The model under review builds one solid part; all positions refer to its coordinate system, in mm. Round coordinates to 2 decimals unless told otherwise and drop trailing zeros. Order: outer loops, then holes, each group sorted by start corner. A loop starts at its lowest first (then second) coordinate and runs counter-clockwise, first axis right, second up. Notation, with made-up numbers: (50, 34.25) -> (69, 34.25) arc R25 ccw to (69, 48.25) -> close; hole circle Ø3 at (37.5, -13.75). An arc over 180 degrees is marked (long way). Put each result on its own line as item: value. Start each with the question number.
Autodesk Inventor part; units mm, degrees
ref_plane "YZ Plane" through (0, 0, 0) normal (1, 0, 0) x (0, 1, 0)
ref_plane "XZ Plane" through (0, 0, 0) normal (0, 1, 0) x (-1, 0, 0)
ref_plane "XY Plane" through (0, 0, 0) normal (0, 0, 1) x (1, 0, 0)
sketch "Эскиз1" plane through (0, 0, 0) normal (0, 0, 1) x (1, 0, 0)
  line L0 (-40, 0) -> (40, 0) construction
  line L1 (-40, -15) -> (40, -15)
  line L2 (40, 15) -> (-40, 15)
  arc A0 (-40, 15) -> (-40, -15) centre (-40, 0) ccw
  arc A1 (40, -15) -> (40, 15) centre (40, 0) ccw
  circle A2 centre (0, 0) radius 12.5
  circle A3 centre (0, 0) radius 6
  circle A4 centre (40, 0) radius 5
  circle A5 centre (-40, 0) radius 5
  dimension "d2" = 80
  dimension "d3" = 30
  dimension "d4" = 25
  dimension "d5" = 12
  dimension "d6" = 10
  dimension "d7" = 10
extrude "Выдавливание1" add sketch "Эскиз1" along normal blind 8 contours A0 L2 A1 L1 | A2 | A4 | A5
extrude "Выдавливание2" cut sketch "Эскиз1" along normal blind 8 contours A4 | A5
extrude "Выдавливание3" add sketch "Эскиз1" along normal blind 20 contours A2
properties part number "lab3_1" material "Свинец"
Q1. Take a section at B-B on x = 0. Give the boundary of the cut face in (y, z), and give its area (3 significant figures).
Q2. Draft analysis for pull direction Y (two halves, no side actions). For faces 1 (the face through (-1, -15, 4)), 2 (the face through (35, 0, 4)), 3 (the face through (11.923, -3.755, 13.916)), state which applies: +Y half, -Y half, draft (parallel to the pull), parting line (faces both ways), or undercut.
Q3. Take a section at A-A on y = 0. Give the boundary of the cut face in (x, z).
Q4. Wall thickness on probe 1 along Y at (x, z) = (0, 5.5); probe 2 along Y at (x, z) = (40, 2.5); probe 3 along X at (y, z) = (-1.5, 4): over which ranges is each line inside the solid? List them lowest first. Write a range as [from, to].
Q5. Take a section at D-D on x = -18.5. Give the boundary of the cut face in (y, z), and give its area (3 significant figures).
Q6. Take a section at C-C on z = 14.75. Give the boundary of the cut face in (x, y).
Q7. Clearance check with flat-ended pins moving along their axes: pin 1 Ø1.5 at (x, y) = (-30.5, -5) entering from +Z; pin 2 Ø4 at (y, z) = (-7.5, 13) entering from -X (3 decimals); pin 3 Ø1 at (y, z) = (9.5, 9.5) entering from -X. State where each tip first meets the part, or that it passes through.
Calculated:
1. outline: (-15, 0) -> (-6, 0) -> (-6, 20) -> (-12.5, 20) -> (-12.5, 8) -> (-15, 8) -> close; (6, 0) -> (15, 0) -> (15, 8) -> (12.5, 8) -> (12.5, 20) -> (6, 20) -> close
1. area: 300 mm²
2. face 1: -Y half
2. face 2: undercut
2. face 3: parting line
3. outline: (-55, 0) -> (-45, 0) -> (-45, 8) -> (-55, 8) -> close; (-35, 0) -> (-6, 0) -> (-6, 20) -> (-12.5, 20) -> (-12.5, 8) -> (-35, 8) -> close; (6, 0) -> (35, 0) -> (35, 8) -> (12.5, 8) -> (12.5, 20) -> (6, 20) -> close; (45, 0) -> (55, 0) -> (55, 8) -> (45, 8) -> close
4. probe 1: y = [-15, -6], [6, 15]
4. probe 2: y = [-15, -5], [5, 15]
4. probe 3: x = [-54.92, -44.77], [-35.23, -5.81], [5.81, 35.23], [44.77, 54.92]
5. outline: (-15, 0) -> (15, 0) -> (15, 8) -> (-15, 8) -> close
5. area: 240 mm²
6. outline: circle Ø25 at (0, 0); hole circle Ø12 at (0, 0)
7. pin 1: stops at z = 8
7. pin 2: stops at x = -11.225
7. pin 3: stops at x = -8.67
